Model file for the job. Use its own axes, mm. A direction names the side the tool comes from. Coordinates: 2 decimals unless noted, no trailing zeros. Write each loop counter-clockwise with the first axis right and the second up, starting at its lowest first coordinate (ties: lowest second). Pieces come first, ordered by that corner, then holes. Notation, with made-up numbers: (16, -32.5) -> (75, -32.5) arc R23 cw to (75, -7.5) -> close; hole circle Ø2 at (45.5, -39). An arc over 180 degrees is marked (long way). Answer as a JSON object with one key per item and string values. Group by question number.
from build123d import *

# Parameters (mm, degrees)
F1_DEPTH = 8


with BuildPart() as f1:
    # F0 (on Front) → F1 (new body)
    with BuildSketch(Plane.XZ):
        with BuildLine():
            Line((18.3469315144, 5.9655109539), (20.9992617956, 21.3784781252))
            ThreePointArc((20.9992617956, 21.3784781252), (0.1249015369, 42.2834629222), (-20.9966564617, 21.6282676124))
            Line((-20.9966564617, 21.6282676124), (-20.9966564617, -1.7508006927))
            add(Edge.make_bspline(
                [(-21.0375948323, -1.8897012773), (-21.0239493062, -1.8434000403), (-21.0103048446, -1.7970993287), (-20.9966564617, -1.7508006927)],
                knots=[0.9931808639, 0.9931808639, 0.9931808639, 0.9931808639, 1, 1, 1, 1], degree=3))
            add(Edge.make_bspline(
                [(-23.311607346, -7.9496343517), (-22.2567283878, -6.0202595283), (-21.6461032363, -3.9544580126), (-21.0375948323, -1.8897012773)],
                knots=[0.6890883985, 0.6890883985, 0.6890883985, 0.6890883985, 0.9931808639, 0.9931808639, 0.9931808639, 0.9931808639], degree=3))
            add(Edge.make_bspline(
                [(-28.2252900615, -13.3057116458), (-26.0825142955, -11.9279404299), (-24.4419956281, -10.0171158148), (-23.311607346, -7.9496343517)],
                knots=[0.3632286809, 0.3632286809, 0.3632286809, 0.3632286809, 0.6890883985, 0.6890883985, 0.6890883985, 0.6890883985], degree=3))
            add(Edge.make_bspline(
                [(-36.6373678698, -16.5920499712), (-33.6263584299, -15.7149316784), (-30.6137952155, -14.8414830049), (-28.2252900615, -13.3057116458)],
                knots=[0, 0, 0, 0, 0.3632286809, 0.3632286809, 0.3632286809, 0.3632286809], degree=3))
            Line((-36.6373678698, -16.5920499712), (-60, -16.5920499712))
            Line((-60, -16.5920499712), (-60, -31.5920499712))
            Line((-60, -31.5920499712), (60, -31.5920499712))
            Line((60, -31.5920499712), (60, -16.5920499712))
            Line((60, -16.5920499712), (9.6341452579, -16.5920499712))
            ThreePointArc((9.6341452579, -16.5920499712), (-0.638590167, -11.7618423985), (-5.9901359502, -1.7508006927))
            Line((-5.9901359502, -1.7508006927), (-5.9901359502, 1.160080022))
            Line((-5.9901359502, 1.160080022), (-5.9901359502, 20.940455724))
            ThreePointArc((-5.9901359502, 20.940455724), (-6, 21.2843616682), (-5.9901359502, 21.6282676124))
            ThreePointArc((-5.9901359502, 21.6282676124), (0, 27.2843616682), (5.9901359502, 21.6282676124))
            Line((5.9901359502, 21.6282676124), (5.9992617956, 21.6282676124))
            Line((5.9992617956, 21.6282676124), (5.9992617956, 21.3784781252))
            ThreePointArc((5.9992617956, 21.3784781252), (6, 21.2843616682), (5.9992617956, 21.1902452111))
            Line((5.9992617956, 21.1902452111), (5.9992617956, 8.1959165921))
            Line((5.9992617956, 8.1959165921), (6.0103126276, 8.1929609357))
            ThreePointArc((6.0103126276, 8.1929609357), (6.0047534058, 8.1727079211), (5.9992617956, 8.1524364691))
            ThreePointArc((5.9992617956, 8.1524364691), (10.4711267055, 0.4310945937), (18.1705571166, 4.9405809808))
            Line((18.1705571166, 4.9405809808), (18.3469315144, 5.9655109539))
        make_face()
        Polygon((-20.9966564617, -1.7508006927), (-20.9966564617, 21.6282676124), (-21.0130866617, -1.7508006927), align=None)
        with BuildLine():
            ThreePointArc((18.1705571166, 4.9405809808), (18.2799498035, 5.449396835), (18.3469315144, 5.9655109539))
            Line((18.3469315144, 5.9655109539), (18.1705571166, 4.9405809808))
        make_face()
        with BuildLine():
            add(Edge.make_bspline(
                [(-21.0375948323, -1.8897012773), (-21.0239493062, -1.8434000403), (-21.0103048446, -1.7970993287), (-20.9966564617, -1.7508006927)],
                knots=[0.9931808639, 0.9931808639, 0.9931808639, 0.9931808639, 1, 1, 1, 1], degree=3))
            Line((-20.9966564617, -1.7508006927), (-21.0130866617, -1.7508006927))
            ThreePointArc((-21.0130866617, -1.7508006927), (-21.0252049482, -1.8202749459), (-21.0375948323, -1.8897012773))
        make_face()
        with BuildLine():
            add(Edge.make_bspline(
                [(-28.2252900615, -13.3057116458), (-26.0825142955, -11.9279404299), (-24.4419956281, -10.0171158148), (-23.311607346, -7.9496343517)],
                knots=[0.3632286809, 0.3632286809, 0.3632286809, 0.3632286809, 0.6890883985, 0.6890883985, 0.6890883985, 0.6890883985], degree=3))
            ThreePointArc((-23.311607346, -7.9496343517), (-25.4958010969, -10.8778007993), (-28.2252900615, -13.3057116458))
        make_face()
        with BuildLine():
            Line((5.9992617956, 21.3784781252), (5.9992617956, 21.1902452111))
            ThreePointArc((5.9992617956, 21.1902452111), (6, 21.2843616682), (5.9992617956, 21.3784781252))
        make_face()
        with BuildLine():
            ThreePointArc((5.9901359502, 21.6282676124), (5.9959997727, 21.5034203961), (5.9992617956, 21.3784781252))
            Line((5.9992617956, 21.3784781252), (5.9992617956, 21.6282676124))
            Line((5.9992617956, 21.6282676124), (5.9901359502, 21.6282676124))
        make_face()
        with BuildLine():
            Line((-5.9901359502, 20.940455724), (-5.9901359502, 21.6282676124))
            ThreePointArc((-5.9901359502, 21.6282676124), (-6, 21.2843616682), (-5.9901359502, 20.940455724))
        make_face()
    extrude(amount=F1_DEPTH)


solid = f1.part
(1) Wall check: probe 1 along X at (y, z) = (-0.25, 6); probe 2 along Z at (x, y) = (-40, -0.25); probe 3 along Z at (x, y) = (10, -1). Give the ranges that are in metal, low to high.
(2) Pin check, flat tips, straight feed: pin 1 (10 mm diameter, centred on x = -16, z = 14, fed in from +Y); pin 2 (3 mm diameter, centred on x = 34.5, y = -2, fed in from +Z); pin 3 (2.5 mm diameter, centred on y = -6, z = 15.5, fed in from +X); pin 4 (12 mm diameter, centred on x = 46.5, z = -5, fed in from -Y). Stop position of each tip, or through.
(3) Cut at A-A on x = 0. List the corners of the cut face in (y, z).
(4) Pull direction Z, two halves, no side cores. Call faces 1 (the face through (-25.46, -3.94, -10.84)), 2 (the face through (-1, 0, -19)), 3 (the face through (19.655, -3.944, 13.564)), 4 (the face through (-1, -4, -31.592)): released by +Z, released by -Z, zero draft, split by the parting line, or undercut.
(5) Cut at B-B on z = 1.5. List the corners of the cut face in (x, y), plus the area to 3 significant figures.
(6) 3-axis set-ups, long thin cutter, end or side, ignore diameter. For faces 5 (the face through (-60, -4, -24)), 6 (the face through (-48, -4, -16.592)), 7 (the face through (-0.521, -3.944, -11.873)), 8 (the face through (5.999, -4, 15)): which of +Z, -Z, +X, -X, +Y, -Y reach the whole face in a straight line?
(7) Cut at C-C on x = 43. List the corners of the cut face in (y, z).
Results found:
{
 "1": {"probe 1": "x = -21.01 to -5.99, 5.8 to 18.35", "probe 2": "z = -31.59 to -16.59", "probe 3": "z = -31.59 to -16.59, 0.58 to 39.75"},
 "2": {"pin 1": "stops at y = 0", "pin 2": "stops at z = -16.59", "pin 3": "stops at x = 20.2", "pin 4": "passes through"},
 "3": {"outline": "(-8, -31.59) -> (0, -31.59) -> (0, -12.34) -> (-8, -12.34) -> close; (-8, 27.28) -> (0, 27.28) -> (0, 42.28) -> (-8, 42.28) -> close"},
 "4": {"face 1": "released by +Z", "face 2": "zero draft", "face 3": "undercut", "face 4": "released by -Z"},
 "5": {"outline": "(-21.01, -8) -> (-5.99, -8) -> (-5.99, 0) -> (-21.01, 0) -> close; (8.28, -8) -> (15.88, -8) -> (15.88, 0) -> (8.28, 0) -> close", "area": "181 mm²"},
 "6": {"face 5": "+Z, -Z, -X, +Y, -Y", "face 6": "+Z, -X, +Y, -Y", "face 7": "+X, +Y, -Y", "face 8": "+Y, -Y"},
 "7": {"outline": "(-8, -31.59) -> (0, -31.59) -> (0, -16.59) -> (-8, -16.59) -> close"}
}
